The model under review builds one solid part; all positions refer to its coordinate system, in mm. Face numbers are marked on the shaded views. A direction names the side the tool comes from. Round coordinates to 2 decimals unless told otherwise and drop trailing zeros. Write each loop counter-clockwise with the first axis right and the second up, starting at its lowest first coordinate (ties: lowest second). Pieces come first, ordered by that corner, then holes. Notation, with made-up numbers: M 84.5,-10.75 L 117.5,-10.75 A19 cw 117.5,16.25 Z; hole C 77,84 d11. An arc over 180 degrees is marked long. Write item = value, one per line. Start each with the question number.
Item 1: Take a section at D-D, the plane y = 0.7. Give the boundary of the cut face in (x, z), plus the area to 3 significant figures.
Item 2: Take a section at A-A, the plane y = 0. Give the boundary of the cut face in (x, z) (3 decimals).
Item 3: Take a section at B-B, the plane x = -1.75. Give the boundary of the cut face in (y, z) (3 decimals).
Item 4: Tool access review of the marked faces 1, 2, 3 and 4: name each direction out of +Z, -Z, +X, -X, +Y, -Y from which nothing blocks a thin tool from reaching the whole face with its end or side.
Item 5: For pin 1 Ø1 at (x, z) = (-1.5, -3) entering from +Y, flat-tipped, find the tip position at first contact; note if it passes through.
Item 6: Take a section at C-C, the plane z = 0.75. Give the boundary of the cut face in (x, y) (3 decimals), plus the area to 3 significant figures.
Item 7: To check wall thickness, follow line 1 along Z through (x, y) = (4, -0.05); line 2 along X through (y, z) = (-0.3, -1.75); line 3 along Z through (x, y) = (-2.5, 0.85). State the ranges of each line that lie inside material, in increasing order.
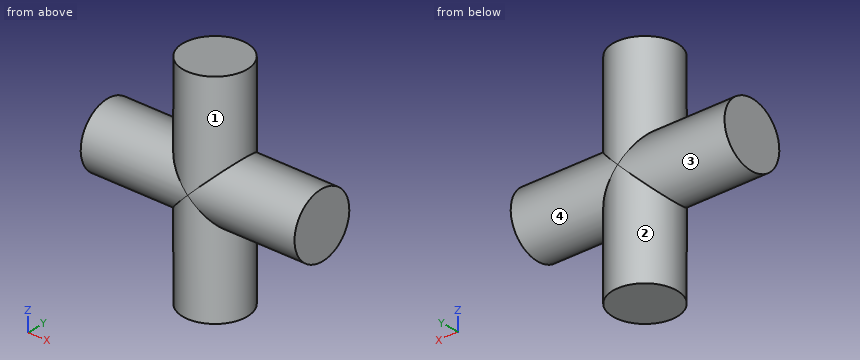
from build123d import *

# Parameters (mm, degrees)
SKETCH1_R           = 1.475
BOSS_EXTRUDE1_DEPTH = 5
SKETCH2_R           = 1.475
BOSS_EXTRUDE2_DEPTH = 5


with BuildPart() as part:
    # Sketch1 → Boss-Extrude1 (new body, symmetric)
    with BuildSketch(Plane.XY):
        Circle(SKETCH1_R)
    extrude(amount=BOSS_EXTRUDE1_DEPTH, both=True)

    # Sketch2 → Boss-Extrude2 (add, symmetric)
    with BuildSketch(Plane(origin=(0, 0, 0), x_dir=(0, 0, -1), z_dir=(1, 0, 0))):
        Circle(SKETCH2_R)
    extrude(amount=BOSS_EXTRUDE2_DEPTH, both=True)


solid = part.part
Response values:
q1.outline = M -5,-1.3 L -1.3,-1.3 L -1.3,-5 L 1.3,-5 L 1.3,-1.3 L 5,-1.3 L 5,1.3 L 1.3,1.3 L 1.3,5 L -1.3,5 L -1.3,1.3 L -5,1.3 Z
q1.area = 45.2 mm2
q2.outline = M -5,-1.475 L -1.475,-1.475 L -1.475,-5 L 1.475,-5 L 1.475,-1.475 L 5,-1.475 L 5,1.475 L 1.475,1.475 L 1.475,5 L -1.475,5 L -1.475,1.475 L -5,1.475 Z
q3.outline = C 0,0 d2.95
q4.face_1 = +Z
q4.face_2 = -Z
q4.face_3 = -X
q4.face_4 = +X
q5.pin_1 = 1.08
q6.outline = M -5,-1.27 L -0.75,-1.27 A1.475 ccw 0.75,-1.27 L 5,-1.27 L 5,1.27 L 0.75,1.27 A1.475 ccw -0.75,1.27 L -5,1.27 Z
q6.area = 25.8 mm2
q7.line_1 = -1.47 to 1.47
q7.line_2 = -1.44 to 1.44
q7.line_3 = -1.21 to 1.21
